Input: dimensioned drawing with shaded views. Units: mm. Origin: part minimum x, y, z. Round coordinates to 2 decimals unless told otherwise and drop trailing zeros. Loops run counter-clockwise (first coordinate to the right, second up) from the corner with the lowest first, then second, coordinate; pieces in that order, holes last. Notation, with made-up numbers: M 60,59.25 L 108,59.25 A20 ccw 108,64.25 Z; hole C -31.5,17.5 d9. An arc over 180 degrees is marked long. Answer as CSV lines item,"result". Start each with the question number.
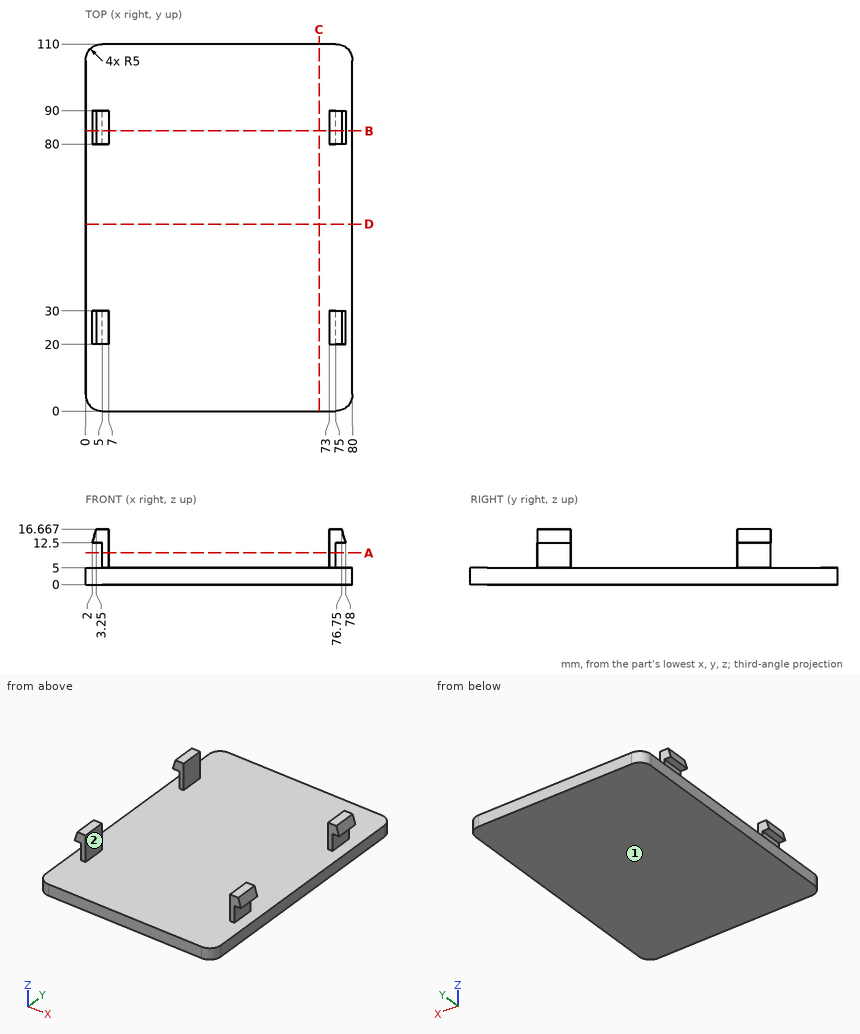
1) Ray query, line 1 along Y through (x, z) = (77, 13); line 2 along Z through (x, y) = (37, 27.5). Return the intervals inside material, ascending.
2) Section C-C, the plane x = 70. Return loops of the section in (y, z), and give its area (3 significant figures).
3) Contact query for flat-ended pins moving along their axis: pin 1 Ø5.5 at (x, z) = (75.5, 12) entering from +Y; pin 2 Ø3 at (y, z) = (23.5, 11.5) entering from -X; pin 3 Ø5 at (y, z) = (66.5, 8) entering from +X; pin 4 Ø2.5 at (x, z) = (4, 8) entering from -Y. Output: stop coordinate, or through.
4) Mould query, pull axis X, two halves, no side actions, for the marked faces 1 and 2. Classes: pulls with the +X half, pulls with the -X half, needs draft (parallel to the pull), parting line crosses it, or undercut.
5) Section B-B, the plane y = 84. Return loops of the section in (x, z).
6) Section D-D, the plane y = 56. Return loops of the section in (x, z).
7) Section A-A, the plane z = 9.5. Return loops of the section in (x, y).
Findings below:
1,line 1,"20 to 30, 80 to 90"
1,line 2,"0 to 5"
2,outline,"M 0,0 L 110,0 L 110,5 L 0,5 Z"
2,area,"550 mm²"
3,pin 1,"y = 90"
3,pin 2,"x = 2"
3,pin 3,"through"
3,pin 4,"y = 20"
4,face 1,"needs draft"
4,face 2,"undercut"
5,outline,"M 0,0 L 80,0 L 80,5 L 75,5 L 75,12.5 L 78,12.5 L 76.75,16.67 L 73,16.67 L 73,5 L 7,5 L 7,16.67 L 3.25,16.67 L 2,12.5 L 5,12.5 L 5,5 L 0,5 Z"
6,outline,"M 0,0 L 80,0 L 80,5 L 0,5 Z"
7,outline,"M 5,20 L 7,20 L 7,30 L 5,30 Z; M 5,80 L 7,80 L 7,90 L 5,90 Z; M 73,20 L 75,20 L 75,30 L 73,30 Z; M 73,80 L 75,80 L 75,90 L 73,90 Z"
